Check sheet for the modelled part. Datum: model origin and axes. Units: mm. A direction names the side the tool comes from. Round coordinates to 2 decimals unless told otherwise and drop trailing zeros. Loops run counter-clockwise (first coordinate to the right, second up) from the corner with the lowest first, then second, coordinate; pieces in that order, holes last. Notation, with made-up numbers: (75.5, 52.25) - (106.5, 52.25) arc R21 cw to (106.5, 62.25) - close; hole circle Ø3 at (-14.5, 54). An arc over 180 degrees is marked (long way). Answer in a Markdown table with one row per item. Add a question column.
(1) Thickness scan on line 1 along X through (y, z) = (88, 81); line 2 along Z through (x, y) = (21, 50); line 3 along Y through (x, z) = (39, 83.5). Record the ranges inside material, lowest first.
(2) Cross-section at D-D on y = 90. Enter the section's corners in (x, z).
(3) Cross-section at C-C on z = 54.5. Enter the section's corners in (x, y).
(4) Cross-section at B-B on x = 30. Enter the section's corners in (y, z), then the cut area to 3 significant figures.
(5) Mould release check, pull along Y, two halves, no side actions. Record for faces 1 (the cylindrical face through (214.65, 51.099, 119.988)), 2 (the flat face through (240, 49, 34)), 3 (the cylindrical face through (215.35, 46.095, 99.745)), 4 (the flat face through (118, 100, 27)): +Y half, -Y half, draft (parallel to the pull), parting line (faces both ways), or undercut.
(6) Access from +Z, -Z, +X, -X, +Y, -Y to the whole of each face (thin tool, end or side, straight path). Record for faces 5 (the flat face through (118, 0, 28)), 6 (the flat face through (50, 28, 96)).
(7) Cross-section at A-A on y = 50. Enter the section's corners in (x, z), then the cut area to 3 significant figures.
(8) Gauge pin test, flat ends, axial feed: pin 1 (1 mm diameter, centred on x = 41.5, y = 44.5, fed in from +Z); pin 2 (2 mm diameter, centred on x = 208.5, y = 29.5, fed in from +Z); pin 3 (2 mm diameter, centred on x = 147, y = 34, fed in from +Z). Record the tip position at first contact, or that the pin passes through.
from build123d import *

# Parameters (mm, degrees)
F1_DEPTH = 240
F2_R     = 30
F3_DEPTH = 240
F5_W     = 140
F5_H     = 100
F6_DEPTH = 85.001


with BuildPart() as f1:
    # F0 (on Right) → F1 (new body)
    with BuildSketch(Plane.YZ):
        with BuildLine():
            Line((0, 70), (0, 0))
            Line((0, 0), (100, 0))
            Line((100, 0), (100, 70))
            ThreePointArc((100, 70), (50, 120), (0, 70))
        make_face()
    extrude(amount=F1_DEPTH)

    # F2 (on face) → F3 (cut, through all)
    with BuildSketch(Plane.YZ.offset(240)):
        with Locations((50, 70)):
            Circle(F2_R)
    extrude(amount=-F3_DEPTH, mode=Mode.SUBTRACT)

    # F5 (on offset) → F6 (cut, through all)
    with BuildSketch(Plane(origin=(0, 0, 35), x_dir=(1, 0, 0), z_dir=(0, 0, -1))):
        with Locations((120, -50)):
            Rectangle(F5_W, F5_H)
    extrude(amount=-F6_DEPTH, mode=Mode.SUBTRACT)


solid = f1.part
Answers:
| question | item | result |
|---|---|---|
| 1 | line 1 | x = 0 to 50, 190 to 240 |
| 1 | line 2 | z = 0 to 40, 100 to 120 |
| 1 | line 3 | y = 1.86 to 23.21, 76.79 to 98.14 |
| 2 | outline | (0, 0) - (240, 0) - (240, 100) - (190, 100) - (190, 35) - (50, 35) - (50, 100) - (0, 100) - close |
| 3 | outline | (0, 0) - (50, 0) - (50, 24.31) - (0, 24.31) - close; (0, 75.69) - (50, 75.69) - (50, 100) - (0, 100) - close; (190, 0) - (240, 0) - (240, 24.31) - (190, 24.31) - close; (190, 75.69) - (240, 75.69) - (240, 100) - (190, 100) - close |
| 4 | outline | (0, 0) - (100, 0) - (100, 70) arc R50 ccw to (0, 70) - close; hole circle Ø60 at (50, 70) |
| 4 | area | 8,100 mm^2 |
| 5 | face 1 | parting line |
| 5 | face 2 | draft |
| 5 | face 3 | undercut |
| 5 | face 4 | +Y half |
| 6 | face 5 | +Z, -Z, +X, -X, -Y |
| 6 | face 6 | +Z, +Y, -Y |
| 7 | outline | (0, 0) - (240, 0) - (240, 40) - (190, 40) - (190, 35) - (50, 35) - (50, 40) - (0, 40) - close; (0, 100) - (50, 100) - (50, 120) - (0, 120) - close; (190, 100) - (240, 100) - (240, 120) - (190, 120) - close |
| 7 | area | 10,900 mm^2 |
| 8 | pin 1 | stops at z = 119.75 |
| 8 | pin 2 | stops at z = 116.04 |
| 8 | pin 3 | stops at z = 35 |
